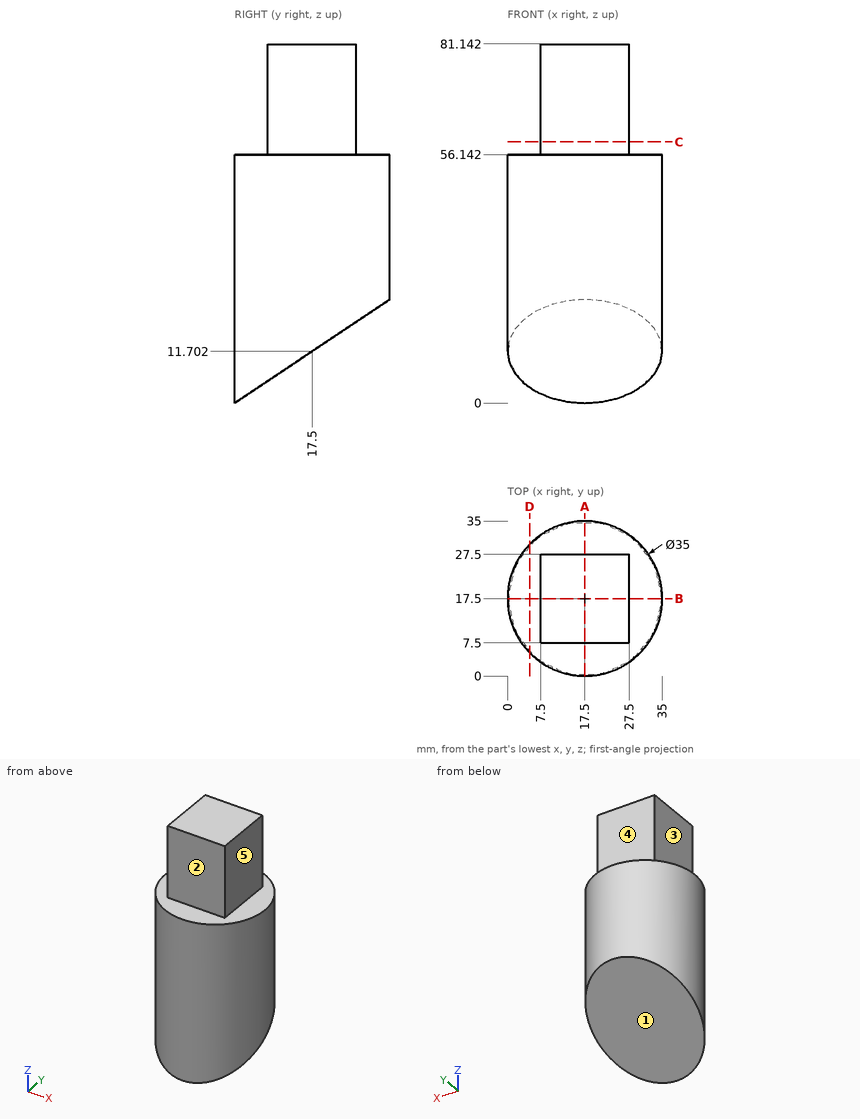
Can you work these out from the drawing? Everything is in mm from the part's minimum corner. A direction names the side the tool comes from. Coordinates: 2 decimals unless noted, no trailing zeros. Loops run counter-clockwise (first coordinate to the right, second up) from the corner with the lowest first, then second, coordinate; pieces in that order, holes last.
1) Imagine slicing it at D-D on x = 5. List the corners of the cut face in (y, z) for me.
2) I need wall thicknesses on probe 1 along X at (y, z) = (24, 72); probe 2 along Y at (x, z) = (17, 44). Which ranges of each line are inside material? Lowest first, please.
3) For pin 1 (16 mm diameter, centred on y = 12.5, z = 69.5, fed in from -X); pin 2 (6 mm diameter, centred on x = 23.5, y = 23, fed in from -Z) (1 decimal); pin 3 (16 mm diameter, centred on y = 18.5, z = 67.5, fed in from +X), each with a flat end and sliding along its axis, tell me the tip position at first contact or that it passes through.
4) Imagine slicing it at A-A on x = 17.5. List the corners of the cut face in (y, z) for me (1 decimal), plus the area to 3 significant figures.
5) Imagine slicing it at B-B on y = 17.5. List the corners of the cut face in (x, z) for me.
6) Imagine slicing it at C-C on z = 59. List the corners of the cut face in (x, y) for me, plus the area to 3 significant figures.
7) Which directions (+Z, -Z, +X, -X, +Y, -Y) give clear straight access to the entire face, cutting with the end or side of a thin tool? Please do the marked faces 1, 2, 3, 4 and 5.
Completed:
1. outline: (5.25, 3.51) - (29.75, 19.89) - (29.75, 56.14) - (5.25, 56.14) - close
2. probe 1: x = 7.5 to 27.5
2. probe 2: y = 0.01 to 34.99
3. pin 1: stops at x = 7.5
3. pin 2: stops at z = 13.4
3. pin 3: stops at x = 27.5
4. outline: (0, 0) - (35, 23.4) - (35, 56.1) - (27.5, 56.1) - (27.5, 81.1) - (7.5, 81.1) - (7.5, 56.1) - (0, 56.1) - close
4. area: 2,060 mm2
5. outline: (0, 11.7) - (35, 11.7) - (35, 56.14) - (27.5, 56.14) - (27.5, 81.14) - (7.5, 81.14) - (7.5, 56.14) - (0, 56.14) - close
6. outline: (7.5, 7.5) - (27.5, 7.5) - (27.5, 27.5) - (7.5, 27.5) - close
6. area: 400 mm2
7. face 1: -Z, +X, -X, +Y
7. face 2: +Z, +X, -X, -Y
7. face 3: +Z, -X, +Y, -Y
7. face 4: +Z, +X, -X, +Y
7. face 5: +Z, +X, +Y, -Y
